from build123d import *

# Parameters (mm, degrees)
SKETCH_1_R           = 4
EXTRUDE_1_DEPTH      = 1.5
SKETCH_1_3_R         = 3
EXTRUDE_2_DEPTH      = 11
CUT_EXTRUDE_START    = 10.1
SKETCH_1_4_OUTSIDE_W = 13.156
SKETCH_1_4_OUTSIDE_H = 13.156
SKETCH_1_4_OUTSIDE_R = 2.8
CUT_EXTRUDE_1_DEPTH  = 0.6


with BuildPart() as part:
    # 草图1 → 凸台-拉伸1 (new body)
    with BuildSketch(Plane.XY):
        with Locations((0.365715483, 0.182857742)):
            Circle(SKETCH_1_R)
    extrude(amount=EXTRUDE_1_DEPTH)

    # 草图1<3> → 凸台-拉伸2 (add)
    with BuildSketch(Plane.XY):
        with Locations((0.365715483, 0.182857742)):
            Circle(SKETCH_1_3_R)
    extrude(amount=EXTRUDE_2_DEPTH)

    # 草图1<4> outside → 切除-拉伸1 (cut)
    with BuildSketch(Plane.XY.offset(CUT_EXTRUDE_START)):
        with Locations((0.366, 0.183)):
            Rectangle(SKETCH_1_4_OUTSIDE_W, SKETCH_1_4_OUTSIDE_H)
        with Locations((0.365715483, 0.182857742)):
            Circle(SKETCH_1_4_OUTSIDE_R, mode=Mode.SUBTRACT)
    extrude(amount=-CUT_EXTRUDE_1_DEPTH, mode=Mode.SUBTRACT)


solid = part.part
For this review, take the finished solid that the model builds, in its own axes (mm). A direction names the side the tool comes from. Coordinates: 2 decimals unless noted, no trailing zeros. Loops run counter-clockwise (first coordinate to the right, second up) from the corner with the lowest first, then second, coordinate; pieces in that order, holes last. Notation, with made-up numbers: (53, 49) - (102, 49) arc R25 ccw to (102, 83) - close; hole circle Ø9 at (83.5, -17.75). An arc over 180 degrees is marked (long way). Use a Markdown table: item, result. Add a question column.
Item 1: Mouldability with a two-part tool opening along Z and no side actions: class faces 1 (the face through (3.036, 1.024, 9.804)), 2 (the face through (-0.285, -2.746, 5.444)), 3 (the face through (0, 0, 0)), 4 (the face through (2, 3, 1.5)) as pulls with the +Z half, pulls with the -Z half, needs draft (parallel to the pull), parting line crosses it, or undercut.
Item 2: We need section A-A (x = 0.25). Give the boundary of the cut face in (y, z), and give its area (3 significant figures).
Item 3: We need section C-C (z = 1.25). Give the boundary of the cut face in (x, y), and give its area (3 significant figures).
Item 4: Insertion check: pin 1 Ø2 at (x, z) = (-1.5, 9) entering from +Y; pin 2 Ø1.5 at (x, z) = (1, 2.5) entering from +Y; pin 3 Ø4 at (x, z) = (3, 5) entering from -Y. Each pin has a flat end and moves straight along its axis. Give the tip position at first contact, or say it passes through.
Item 5: For line 1 (Z direction, x = 3, y = 1.25); line 2 (Z direction, x = 3.75, y = -0.25); line 3 (X direction, y = 0.75, z = 10.75), list the stretches that pass through material, from the lowest coordinate up.
Item 6: Tool access review of faces 5 (the face through (-0.285, -2.746, 10.544)), 6 (the face through (0, 0, 11)): name each direction out of +Z, -Z, +X, -X, +Y, -Y from which nothing blocks a thin tool from reaching the whole face with its end or side.
Item 7: We need section D-D (z = 3.5). Give the boundary of the cut face in (x, y).
Item 8: We need section B-B (y = 2.25). Give the boundary of the cut face in (x, z).
Results list:
| question | item | result |
|---|---|---|
| 1 | face 1 | undercut |
| 1 | face 2 | needs draft |
| 1 | face 3 | pulls with the -Z half |
| 1 | face 4 | pulls with the +Z half |
| 2 | outline | (-3.82, 0) - (4.18, 0) - (4.18, 1.5) - (3.18, 1.5) - (3.18, 9.5) - (2.98, 9.5) - (2.98, 10.1) - (3.18, 10.1) - (3.18, 11) - (-2.81, 11) - (-2.81, 10.1) - (-2.61, 10.1) - (-2.61, 9.5) - (-2.81, 9.5) - (-2.81, 1.5) - (-3.82, 1.5) - close |
| 2 | area | 68.7 mm^2 |
| 3 | outline | circle Ø8 at (0.37, 0.18) |
| 3 | area | 50.3 mm^2 |
| 4 | pin 1 | stops at y = 3.06 |
| 4 | pin 2 | stops at y = 3.18 |
| 4 | pin 3 | stops at y = -2.75 |
| 5 | line 1 | z = 0 to 9.5, 10.1 to 11 |
| 5 | line 2 | z = 0 to 1.5 |
| 5 | line 3 | x = -2.58 to 3.31 |
| 6 | face 5 | +Z |
| 6 | face 6 | +Z, +X, -X, +Y, -Y |
| 7 | outline | circle Ø6 at (0.37, 0.18) |
| 8 | outline | (-3.06, 0) - (3.79, 0) - (3.79, 1.5) - (2.54, 1.5) - (2.54, 9.5) - (2.25, 9.5) - (2.25, 10.1) - (2.54, 10.1) - (2.54, 11) - (-1.81, 11) - (-1.81, 10.1) - (-1.52, 10.1) - (-1.52, 9.5) - (-1.81, 9.5) - (-1.81, 1.5) - (-3.06, 1.5) - close |
